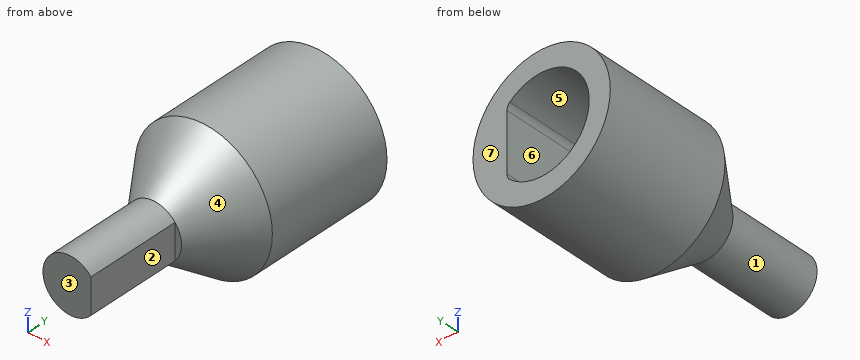
```python
from build123d import *

# Parameters (mm, degrees)
SKETCH1_R               = 8
BOSS_EXTRUDE1_DEPTH     = 10
SKETCH3_W               = 0.75
SKETCH3_H               = 11
CUT_EXTRUDE1_DEPTH      = 12
CUT_EXTRUDE1_DEPTH_BACK = 12
FILLET2_R               = 1
FILLET3_R               = 1


with BuildPart() as part:
    # Sketch1 → Boss-Extrude1 (new body)
    with BuildSketch(Plane(origin=(0, 0, 0), x_dir=(1, 0, 0), z_dir=(0, 1, 0))):
        Circle(SKETCH1_R)
        with BuildLine():
            Line((4.036363636, -0.000130644), (4.036363636, 3.809234647))
            ThreePointArc((4.036363636, 3.809234647), (-5.55, 0), (4.036363636, -3.809234647))
            Line((4.036363636, -3.809234647), (4.036363636, -0.000130644))
        make_face(mode=Mode.SUBTRACT)
    extrude(amount=BOSS_EXTRUDE1_DEPTH)

    # Sketch2 → Revolve1 (revolve)
    with BuildSketch(Plane.XY):
        Polygon((8, 0), (8, -5), (3.175, -11.473666382), (3.175, -22.473666382), (0, -22.473666382), (0, 0), align=None)
    revolve(axis=Axis((0, -22.473666382, 0), (0, -1, 0)))

    # Sketch3 → Cut-Extrude1 (cut, two sides)
    with BuildSketch(Plane.XY) as cut_extrude1_sk:
        with Locations((2.8, -16.973666382)):
            Rectangle(SKETCH3_W, SKETCH3_H)
    extrude(amount=CUT_EXTRUDE1_DEPTH, mode=Mode.SUBTRACT)
    extrude(cut_extrude1_sk.sketch, amount=-CUT_EXTRUDE1_DEPTH_BACK, mode=Mode.SUBTRACT)

    # Fillet2
    fillet2_edges = [part.edges().sort_by_distance(p)[0] for p in [
        (4.036363636, 5, -3.809234647),
    ]]
    fillet(fillet2_edges, radius=FILLET2_R)

    # Fillet3
    fillet3_edges = [part.edges().sort_by_distance(p)[0] for p in [
        (4.036363636, 5, 3.809234647),
    ]]
    fillet(fillet3_edges, radius=FILLET3_R)


solid = part.part
```
Part model, mm, in its own coordinate system. Face numbers are marked on the shaded views. A direction names the side the tool comes from. Round coordinates to 2 decimals unless told otherwise and drop trailing zeros. Loops run counter-clockwise (first coordinate to the right, second up) from the corner with the lowest first, then second, coordinate; pieces in that order, holes last.
Item 1: Drop flat-ended pins along their axis: P1, Ø5, axis at x = 0.5, z = 1, coming from the +Y side; P2, Ø1.5, axis at y = -8, z = 3.5, coming from the -X side; P3, Ø6, axis at x = 2.5, z = -1, coming from the +Y side; P4, Ø1.5, axis at y = -7.5, z = 6, coming from the -X side. Give the stop position or say it passes through.
Item 2: 3-axis set-ups, long thin cutter, end or side, ignore diameter. For the marked faces 1, 2 and 3: which of +Z, -Z, +X, -X, +Y, -Y reach the whole face in a straight line?
Item 3: Cut at D-D, the plane y = -13.5. Give the cut face in (x, z) (3 decimals), then the cut area to 3 significant figures.
Item 4: Drill centre lines: line 1 (Z direction, x = 0, y = 3.25); line 2 (Y direction, x = 2.75, z = -1.5); line 3 (Y direction, x = 1.5, z = -2). Where is each one in solid material? Low to high.
Item 5: Cut at B-B, the plane y = 5. Give the cut face in (x, z).
Item 6: Cut at A-A, the plane x = 0. Give the cut face in (y, z) (3 decimals), then the cut area to 3 significant figures.
Item 7: Cut at C-C, the plane z = 0. Give the cut face in (x, y) (3 decimals).
Item 8: Mould opens along Z. For the marked faces 4, 5, 6 and 7 say: +Z half, -Z half, draft (parallel to the pull), parting line (faces both ways), or undercut.
A:
1. P1: stops at y = 0
1. P2: stops at x = -5.41
1. P3: stops at y = 10
1. P4: stops at x = -3.57
2. face 1: -Y
2. face 2: +Z, -Z, +X, -Y
2. face 3: +Z, -Z, +X, -X, -Y
3. outline: (2.425, -2.049) - (2.425, 2.049) arc R3.175 ccw (long way) to start
3. area: 29.6 mm2
4. line 1: z = -8 to -5.55, 5.55 to 8
4. line 2: y = -11.47 to 0
4. line 3: y = -22.47 to 0
5. outline: circle Ø16 at (0, 0); hole (3.7, -4.13) arc R1 ccw to (4.04, -3.39) - (4.04, 3.39) arc R1 ccw to (3.7, 4.13) arc R5.55 ccw (long way) to start
6. outline: (-22.474, -3.175) - (-11.474, -3.175) - (-5, -8) - (10, -8) - (10, -5.55) - (0, -5.55) - (0, 5.55) - (10, 5.55) - (10, 8) - (-5, 8) - (-11.474, 3.175) - (-22.474, 3.175) - close
6. area: 271 mm2
7. outline: (-8, -5) - (-3.175, -11.474) - (-3.175, -22.474) - (2.425, -22.474) - (2.425, -11.474) - (3.175, -11.474) - (8, -5) - (8, 10) - (4.036, 10) - (4.036, 0) - (-5.55, 0) - (-5.55, 10) - (-8, 10) - close
8. face 4: parting line
8. face 5: undercut
8. face 6: undercut
8. face 7: draft
